Check sheet for the modelled part. Datum: model origin and axes. Units: mm. Round coordinates to 2 decimals unless told otherwise and drop trailing zeros. Write each loop counter-clockwise with the first axis right and the second up, starting at its lowest first coordinate (ties: lowest second). Pieces come first, ordered by that corner, then holes. Notation, with made-up numbers: (-7, 53) - (3, 53) arc R29 ccw to (3, 78) - close; hole circle Ø10 at (66, 82). An arc over 180 degrees is marked (long way). Use one line per item in the form item = value. Start each with the question number.
1) Section check A-A (z = -79). Record the boundary of the cut face in (x, y).
2) Gauge pin test, flat ends, axial feed: P1, Ø2.5, axis at x = 190.5, y = 5, coming from the +Z side; P2, Ø1, axis at y = 5.5, z = -94, coming from the -X side; P3, Ø2.5, axis at y = 5, z = -189, coming from the +X side. Record the tip position at first contact, or that the pin passes through.
3) Draft check along X on faces 1 (the face through (190.361, 1.972, -190.245)), 2 (the face through (187.48, 1.97, -185.33)), 3 (the face through (21, 2, -99)), 4 (the face through (10, 7, -162)). Enter one of: +X half, -X half, draft (parallel to the pull), parting line (faces both ways), or undercut.
4) Section check C-C (y = 2). Record the boundary of the cut face in (x, z).
5) Scan lines: probe 1 along X at (y, z) = (6.75, -157); probe 2 along X at (y, z) = (2.5, -39); probe 3 along Z at (x, y) = (100.5, 4.5). Record each from-to range of solid material in increasing order.
6) Section check B-B (x = 39). Record the boundary of the cut face in (y, z), then the cut area to 3 significant figures.
from build123d import *

# Parameters (mm, degrees)
CROQUIS1_R              = 2.499999999999999
CROQUIS1_R_2            = 2.4999999999999956
CROQUIS1_R_3            = 2.4999999999999982
SALIENTE_EXTRUIR1_DEPTH = 4
CROQUIS2_W              = 158.00000000000003
CROQUIS2_H              = 158
CORTAR_EXTRUIR1_DEPTH   = 10
CROQUIS4_W              = 4.000000000000028
CROQUIS4_H              = 15
CROQUIS4_W_2            = 4
CROQUIS4_H_2            = 14.999999999999972
CROQUIS4_H_3            = 15.000000000000028
CROQUIS4_W_3            = 15.000000000000007
CROQUIS4_H_4            = 4
CROQUIS4_W_4            = 14.999999999999986
CROQUIS4_W_5            = 15.000000000000028
SALIENTE_EXTRUIR2_DEPTH = 3
CORTAR_EXTRUIR2_DEPTH   = 5
REDONDEO1_R             = 7.5


with BuildPart() as part:
    # Croquis1 → Saliente-Extruir1 (new body)
    with BuildSketch(Plane(origin=(0, 0, 0), x_dir=(1, 0, 0), z_dir=(0, 1, 0))):
        Polygon((0, 0), (200, 0), (200, 200), (-2.776e-14, 200), align=None)
        with Locations(Location((14.99999999999995, 185.00000000000003, 0), (0, 0, 270))):
            Circle(CROQUIS1_R, mode=Mode.SUBTRACT)
        with Locations(Location((185, 185.00000000000003, 0), (0, 0, 270))):
            Circle(CROQUIS1_R_2, mode=Mode.SUBTRACT)
        with Locations(Location((185, 15.000000000000055, 0), (0, 0, 270))):
            Circle(CROQUIS1_R_2, mode=Mode.SUBTRACT)
        with Locations(Location((14.999999999999957, 15.000000000000007, 0), (0, 0, 270))):
            Circle(CROQUIS1_R_3, mode=Mode.SUBTRACT)
    extrude(amount=SALIENTE_EXTRUIR1_DEPTH)

    # Croquis2 → Cortar-Extruir1 (cut)
    with BuildSketch(Plane(origin=(0, 4, 0), x_dir=(1, 0, 0), z_dir=(0, 1, 0))):
        with Locations((100.00000000000001, 100.00000000000003)):
            Rectangle(CROQUIS2_W, CROQUIS2_H)
    extrude(amount=-CORTAR_EXTRUIR1_DEPTH, mode=Mode.SUBTRACT)

    # Croquis4 → Saliente-Extruir2 (add)
    with BuildSketch(Plane(origin=(0, 4, 0), x_dir=(1, 0, 0), z_dir=(0, 1, 0))):
        with Locations((10.499999999999982, 130.83333333333337)):
            Rectangle(CROQUIS4_W, CROQUIS4_H)
        with Locations((10.499999999999982, 161.66666666666669)):
            Rectangle(CROQUIS4_W_2, CROQUIS4_H_2)
        with Locations((189.50000000000009, 100.00000000000014)):
            Rectangle(CROQUIS4_W_2, CROQUIS4_H_3)
        with Locations((38.33333333333334, 189.5)):
            Rectangle(CROQUIS4_W_3, CROQUIS4_H_4)
        with Locations((72.91666666666669, 189.5)):
            Rectangle(CROQUIS4_W_4, CROQUIS4_H_4)
        Polygon((8.499999999999995, 107.50000000000003), (12.499999999999995, 107.50000000000003), (12.500000000000005, 92.5), (8.500000000000005, 92.5), align=None)
        with Locations((100, 189.5)):
            Rectangle(CROQUIS4_W_5, CROQUIS4_H_4)
        Polygon((191.5000000000001, 138.33333333333348), (187.50000000000006, 138.33333333333348), (187.50000000000009, 123.33333333333347), (191.50000000000014, 123.33333333333348), align=None)
        Polygon((191.50000000000003, 169.1666666666668), (187.50000000000003, 169.1666666666668), (187.50000000000006, 154.1666666666668), (191.50000000000006, 154.1666666666668), align=None)
        Polygon((169.16666666666666, 187.50000000000009), (154.16666666666666, 187.50000000000009), (154.16666666666666, 191.50000000000009), (169.16666666666663, 191.50000000000009), align=None)
        Polygon((134.58333333333334, 187.50000000000006), (119.58333333333331, 187.50000000000003), (119.58333333333331, 191.50000000000003), (134.58333333333334, 191.50000000000006), align=None)
        Polygon((8.50000000000002, 61.666666666666664), (12.500000000000048, 61.666666666666664), (12.500000000000027, 76.66666666666666), (8.499999999999998, 76.66666666666666), align=None)
        Polygon((8.500000000000071, 30.833333333333325), (12.500000000000073, 30.83333333333335), (12.500000000000055, 45.83333333333332), (8.500000000000055, 45.83333333333332), align=None)
        Polygon((30.83333333333346, 12.500000000000039), (45.83333333333347, 12.500000000000068), (45.83333333333347, 8.500000000000064), (30.833333333333467, 8.500000000000036), align=None)
        Polygon((65.41666666666679, 12.500000000000094), (80.41666666666679, 12.500000000000123), (80.4166666666668, 8.500000000000119), (65.4166666666668, 8.50000000000009), align=None)
        Polygon((107.50000000000013, 12.50000000000015), (92.5000000000001, 12.500000000000123), (92.5000000000001, 8.500000000000119), (107.50000000000013, 8.500000000000146), align=None)
        Polygon((134.58333333333346, 8.500000000000119), (134.58333333333346, 12.500000000000123), (119.58333333333343, 12.50000000000015), (119.58333333333343, 8.500000000000146), align=None)
        Polygon((169.16666666666674, 8.500000000000146), (169.16666666666677, 12.50000000000015), (154.16666666666677, 12.500000000000123), (154.16666666666677, 8.500000000000119), align=None)
        Polygon((191.5000000000001, 45.83333333333345), (191.50000000000014, 30.833333333333464), (187.50000000000014, 30.833333333333464), (187.5000000000001, 45.83333333333345), align=None)
        Polygon((191.5000000000002, 76.66666666666677), (191.50000000000017, 61.666666666666785), (187.5000000000001, 61.666666666666785), (187.50000000000014, 76.66666666666679), align=None)
        with BuildLine():
            ThreePointArc((14.99999999999995, 192.50000000000003), (9.696699141100844, 190.30330085889915), (7.499999999999951, 185.00000000000003))
            ThreePointArc((7.499999999999951, 185.00000000000003), (8.74999999999995, 183.75000000000003), (9.99999999999995, 185.00000000000003))
            ThreePointArc((9.99999999999995, 185.00000000000003), (11.464466094067213, 188.53553390593277), (14.99999999999995, 190.00000000000003))
            ThreePointArc((14.99999999999995, 190.00000000000003), (16.24999999999995, 191.25000000000003), (14.99999999999995, 192.50000000000003))
        make_face()
        with BuildLine():
            ThreePointArc((185.00000000000003, 192.50000000000014), (190.30330085889915, 190.30330085889926), (192.50000000000006, 185.00000000000014))
            ThreePointArc((192.50000000000006, 185.00000000000014), (191.25000000000006, 183.75000000000014), (190.00000000000006, 185.00000000000014))
            ThreePointArc((190.00000000000006, 185.00000000000014), (188.5355339059328, 188.53553390593288), (185.00000000000003, 190.00000000000014))
            ThreePointArc((185.00000000000003, 190.00000000000014), (183.75000000000003, 191.25000000000014), (185.00000000000003, 192.50000000000014))
        make_face()
        with BuildLine():
            ThreePointArc((15.000000000000073, 7.500000000000007), (9.696699141100964, 9.69669914110089), (7.500000000000062, 14.999999999999986))
            ThreePointArc((7.500000000000062, 14.999999999999986), (8.750000000000062, 16.249999999999986), (10.00000000000006, 14.999999999999986))
            ThreePointArc((10.00000000000006, 14.999999999999986), (11.464466094067335, 11.46446609406726), (15.000000000000071, 10.000000000000009))
            ThreePointArc((15.000000000000071, 10.000000000000009), (16.250000000000075, 8.750000000000007), (15.000000000000073, 7.500000000000007))
        make_face()
        with BuildLine():
            ThreePointArc((185.00000000000014, 10.00000000000012), (183.75000000000014, 8.750000000000119), (185.00000000000014, 7.500000000000117))
            ThreePointArc((185.00000000000014, 7.500000000000117), (190.30330085889926, 9.696699141101004), (192.50000000000017, 15.000000000000124))
            ThreePointArc((192.50000000000017, 15.000000000000124), (191.25000000000017, 16.250000000000124), (190.00000000000017, 15.000000000000124))
            ThreePointArc((190.00000000000017, 15.000000000000124), (188.5355339059329, 11.464466094067374), (185.00000000000014, 10.00000000000012))
        make_face()
    extrude(amount=SALIENTE_EXTRUIR2_DEPTH)

    # Croquis5 → Cortar-Extruir2 (cut)
    with BuildSketch(Plane(origin=(0, 4, 0), x_dir=(1, 0, 0), z_dir=(0, 1, 0))):
        Polygon((200, 200), (-2.776e-14, 200), (0, 0), (200, 0), align=None)
        Polygon((192.5, 192.5), (7.500000000000001, 192.49999999999997), (7.500000000000023, 7.5), (192.5, 7.500000000000011), align=None, mode=Mode.SUBTRACT)
    extrude(amount=-CORTAR_EXTRUIR2_DEPTH, mode=Mode.SUBTRACT)

    # Redondeo1
    redondeo1_edges = [part.edges().sort_by_distance(p)[0] for p in [
        (7.500000000000023, 2, -7.5),
        (7.500000000000001, 2, -192.49999999999997),
        (192.5, 2, -192.5),
        (192.5, 2, -7.500000000000011),
    ]]
    fillet(redondeo1_edges, radius=REDONDEO1_R)


solid = part.part
Results are:
q1.outline = (7.5, 0) - (21, 0) - (21, 4) - (7.5, 4) - close; (179, 0) - (192.5, 0) - (192.5, 4) - (179, 4) - close
q2.P1 = -8.82
q2.P2 = 8.5
q2.P3 = 191.98
q3.face_1 = +X half
q3.face_2 = undercut
q3.face_3 = undercut
q3.face_4 = draft
q4.outline = (7.5, -185) arc R7.5 ccw to (15, -192.5) - (185, -192.5) arc R7.5 ccw to (192.5, -185) - (192.5, -15) arc R7.5 ccw to (185, -7.5) - (15, -7.5) arc R7.5 ccw to (7.5, -15) - close; hole circle Ø5 at (15, -185); hole circle Ø5 at (15, -15); hole (21, -179) - (179, -179) - (179, -21) - (21, -21) - close; hole circle Ø5 at (185, -185); hole circle Ø5 at (185, -15)
q5.probe_1 = 8.5 to 12.5, 187.5 to 191.5
q5.probe_2 = 7.5 to 21, 179 to 192.5
q5.probe_3 = -191.5 to -187.5, -12.5 to -8.5
q6.outline = (0, -192.5) - (4, -192.5) - (4, -191.5) - (7, -191.5) - (7, -187.5) - (4, -187.5) - (4, -179) - (0, -179) - close; (0, -21) - (4, -21) - (4, -12.5) - (7, -12.5) - (7, -8.5) - (4, -8.5) - (4, -7.5) - (0, -7.5) - close
q6.area = 132 mm²
